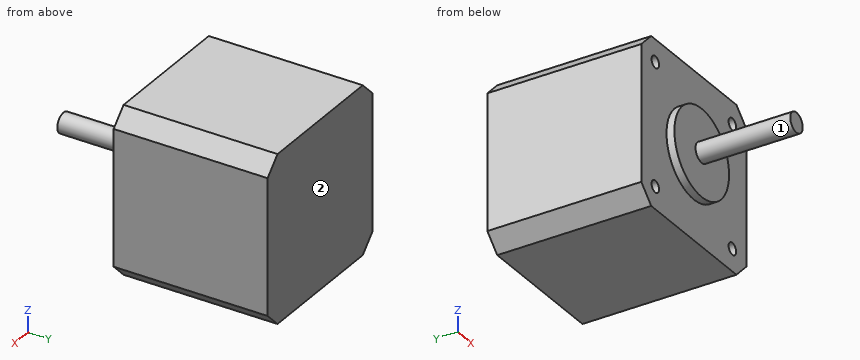
from build123d import *

# Parameters (mm, degrees)
BOX_W        = 42.3
BOX_H        = 39
BOX_DEPTH    = 42.3
CHAMFER_SIZE = 4
SKETCH002_R  = 1.5
POCKET_DEPTH = 5
SKETCH001_R  = 11
PAD001_DEPTH = 2
SKETCH_R     = 2.5
PAD_DEPTH    = 24


with BuildPart() as part:
    # Box → Box (new body)
    with BuildSketch(Plane.XY):
        with Locations((21.15, 19.5)):
            Rectangle(BOX_W, BOX_H)
    extrude(amount=BOX_DEPTH)

    # Chamfer
    chamfer_edges = [part.edges().sort_by_distance(p)[0] for p in [
        (42.3, 19.5, 0),
        (42.3, 19.5, 42.3),
        (0, 19.5, 42.3),
        (0, 19.5, 0),
    ]]
    chamfer(chamfer_edges, length=CHAMFER_SIZE)

    # Sketch002 → Pocket (cut)
    with BuildSketch(Plane.XZ):
        with Locations((5.65, 36.65)):
            Circle(SKETCH002_R)
        with Locations((36.65, 36.65)):
            Circle(SKETCH002_R)
        with Locations((5.65, 5.65)):
            Circle(SKETCH002_R)
        with Locations((36.65, 5.65)):
            Circle(SKETCH002_R)
    extrude(amount=-POCKET_DEPTH, mode=Mode.SUBTRACT)

    # Sketch001 → Pad001 (new body)
    with BuildSketch(Plane.XZ):
        with Locations((21.15, 21.15)):
            Circle(SKETCH001_R)
    extrude(amount=PAD001_DEPTH)

    # Sketch → Pad (new body)
    with BuildSketch(Plane.XZ.offset(2)):
        with Locations((21.15, 21.15)):
            Circle(SKETCH_R)
    extrude(amount=PAD_DEPTH)


solid = part.part
CAD build for the part. Positions are in the model's coordinates, mm. Face numbers are marked on the shaded views. A direction names the side the tool comes from. Give positions to 0.01 mm unless a question says otherwise; leave off trailing zeros. Loops run counter-clockwise (first coordinate to the right, second up) from the corner with the lowest first, then second, coordinate; pieces in that order, holes last. Notation, with made-up numbers: M 31.25,-3.75 L 62.25,-3.75 A9 cw 62.25,3.25 Z; hole C -29.5,84.25 d8. An arc over 180 degrees is marked long. One line per question, with ' | ' between items. Start each with the question number.
1. Flat gauge pins, fed straight in: pin 1 (1.5 mm diameter, centred on x = 36.5, z = 37.5, fed in from -Y); pin 2 (0.9 mm diameter, centred on x = 5.5, z = 36.5, fed in from -Y); pin 3 (4 mm diameter, centred on x = 24.5, z = 10.5, fed in from -Y). Where does each tip first touch, or does it go through?
2. 3-axis set-ups, long thin cutter, end or side, ignore diameter. For the marked faces 1 and 2: which of +Z, -Z, +X, -X, +Y, -Y reach the whole face in a straight line?
3. Saw through at D-D on y = -9. Give the cut face in (x, z).
4. Probe L1, parallel to Z at x = 5.65, y = 1.75; L2, parallel to Z at x = 36, y = 1. List the from-to ranges inside material, lowest first. Write a range as from..to.
5. Saw through at C-C on z = 36.65. Give the cut face in (x, y), plus the area to 3 significant figures.
6. Saw through at A-A on y = 6. Give the cut face in (x, z).
7. Saw through at B-B on x = 36.65. Give the cut face in (y, z).
Result sheet:
1) pin 1: stops at y = 0 | pin 2: stops at y = 5 | pin 3: stops at y = -2
2) face 1: -Y | face 2: +Z, -Z, +X, -X, +Y
3) outline: C 21.15,21.15 d5
4) L1: z = 0..4.15, 7.15..35.15, 38.15..42.3 | L2: z = 0..4.3, 7..35.3, 38..42.3
5) outline: M 0,0 L 4.15,0 L 4.15,5 L 7.15,5 L 7.15,0 L 35.15,0 L 35.15,5 L 38.15,5 L 38.15,0 L 42.3,0 L 42.3,39 L 0,39 Z | area: 1,620 mm^2
6) outline: M 0,4 L 4,0 L 38.3,0 L 42.3,4 L 42.3,38.3 L 38.3,42.3 L 4,42.3 L 0,38.3 Z
7) outline: M 0,0 L 39,0 L 39,42.3 L 0,42.3 L 0,38.15 L 5,38.15 L 5,35.15 L 0,35.15 L 0,7.15 L 5,7.15 L 5,4.15 L 0,4.15 Z
